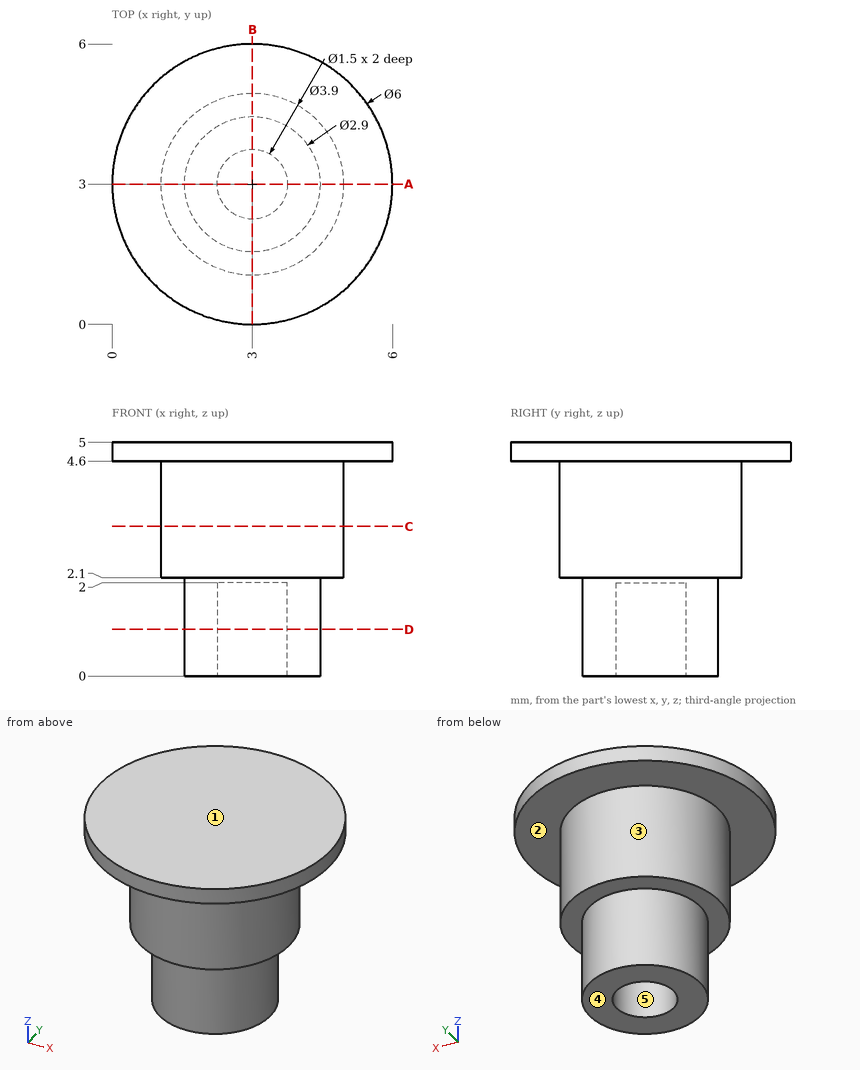
Job drawing, mm, ordinate dimensions from the low corner. One solid piece. A direction names the side the tool comes from. Round coordinates to 2 decimals unless told otherwise and drop trailing zeros. Loops run counter-clockwise (first coordinate to the right, second up) from the corner with the lowest first, then second, coordinate; pieces in that order, holes last. Notation, with made-up numbers: (-10, 9) -> (46, 9) arc R20 ccw to (46, 36) -> close; hole circle Ø1 at (14, 64). An arc over 180 degrees is marked (long way). Use CSV: the item, a comma, the result in double quotes. Start each with the question number.
Q1. Drill centre lines: L1, parallel to X at y = 3, z = 0.55; L2, parallel to Z at x = 2.4, y = 4.55. Where is each one in solid material? Low to high.
Q2. Saw through at C-C on z = 3.2. Give the cut face in (x, y), and give its area (3 significant figures).
Q3. Saw through at A-A on y = 3. Give the cut face in (x, z).
Q4. Which spindle directions (+Z, -Z, +X, -X, +Y, -Y) get a long thin tool onto all of the face, cutting with end or side? Do the marked faces 1 and 2. Say none if no direction does.
Q5. Saw through at D-D on z = 1. Give the cut face in (x, y), and give its area (3 significant figures).
Q6. Mould opens along Y. For the marked faces 3, 4 and 5 say: +Y half, -Y half, draft (parallel to the pull), parting line (faces both ways), or undercut.
Q7. Flat gauge pins, fed straight in: pin 1 Ø0.9 at (x, y) = (3, 3) entering from -Z; pin 2 Ø1 at (y, z) = (4, 4) entering from +X; pin 3 Ø3 at (x, z) = (4.5, 2.5) entering from +Y. Where does each tip first touch, or does it go through?
Solutions:
1,L1,"x = 1.55 to 2.25, 3.75 to 4.45"
1,L2,"z = 2.1 to 5"
2,outline,"circle Ø3.9 at (3, 3)"
2,area,"11.9 mm^2"
3,outline,"(0, 4.6) -> (1.05, 4.6) -> (1.05, 2.1) -> (1.55, 2.1) -> (1.55, 0) -> (2.25, 0) -> (2.25, 2) -> (3.75, 2) -> (3.75, 0) -> (4.45, 0) -> (4.45, 2.1) -> (4.95, 2.1) -> (4.95, 4.6) -> (6, 4.6) -> (6, 5) -> (0, 5) -> close"
4,face 1,"+Z, +X, -X, +Y, -Y"
4,face 2,"-Z"
5,outline,"circle Ø2.9 at (3, 3); hole circle Ø1.5 at (3, 3)"
5,area,"4.84 mm^2"
6,face 3,"parting line"
6,face 4,"draft"
6,face 5,"undercut"
7,pin 1,"stops at z = 2"
7,pin 2,"stops at x = 4.88"
7,pin 3,"stops at y = 4.95"
